Source: CAD feature listing. Evaluate the final solid. Frame: model axes, mm. A direction names the side the tool comes from. Coordinates: 2 decimals unless noted, no trailing zeros. Write each loop counter-clockwise with the first axis right and the second up, starting at its lowest first coordinate (ties: lowest second). Pieces come first, ordered by that corner, then holes. Notation, with made-up numbers: (36.5, -9.75) -> (89.5, -9.75) arc R21 ccw to (89.5, 10.25) -> close; hole circle Ø10 at (-34, 78). An arc over 180 degrees is marked (long way). One line per item, written item: value. Start each with the question number.
1. Mould query, pull axis Y, two halves, no side actions, for faces 3 (the flat face through (-1, 47, -1380)), 4 (the flat face through (1, -50, -1380)), 5 (the flat face through (-48, 0, 0)). Classes: released by +Y, released by -Y, zero draft, split by the parting line, or undercut.
2. First-contact query: P1, Ø1.5, axis at x = 48, z = 41.5, coming from the -Y side. Flat tip, straight axial feed; report the tip coordinate or a pass-through.
3. Section query C-C, the plane x = -18.5. Output: boundary loops of the cut face in (y, z).
4. Access query for faces 1 (the flat face through (49, 1, -2843)), 2 (the flat face through (-47, -1, -1380)). Directions: +Z, -Z, +X, -X, +Y, -Y. A direction counts if a zero-diameter tool reaches every point of the face in a straight line with its end or side. Return the directions, or none.
5. Section query B-B, the plane z = -1213.5. Output: boundary loops of the cut face in (x, y), and give its area (3 significant figures).
6. Section query A-A, the plane y = 20. Output: boundary loops of the cut face in (x, z).
7. Line query: line 1 (Y direction, x = 22, z = -420.5); line 2 (Y direction, x = 44, z = -1473.5). Output: solid intervals per line, ascending.
from build123d import *

# Parameters (mm, degrees)
EXTRUDE_1_DEPTH = 2800
EXTRUDE_2_DEPTH = 3


with BuildPart() as part:
    # Эскиз1 → Бобышка-Вытянуть1 (new body)
    with BuildSketch(Plane.XY):
        with BuildLine():
            Line((-44, 50), (44, 50))
            ThreePointArc((44, 50), (48.242640687, 48.242640687), (50, 44))
            Line((50, 44), (50, -44))
            ThreePointArc((50, -44), (48.242640687, -48.242640687), (44, -50))
            Line((44, -50), (-44, -50))
            ThreePointArc((-44, -50), (-48.242640687, -48.242640687), (-50, -44))
            Line((-50, -44), (-50, 44))
            ThreePointArc((-50, 44), (-48.242640687, 48.242640687), (-44, 50))
        make_face()
        with BuildLine():
            Line((-43, 47), (43, 47))
            ThreePointArc((43, 47), (45.828427125, 45.828427125), (47, 43))
            Line((47, 43), (47, -43))
            ThreePointArc((47, -43), (45.828427125, -45.828427125), (43, -47))
            Line((43, -47), (-43, -47))
            ThreePointArc((-43, -47), (-45.828427125, -45.828427125), (-47, -43))
            Line((-47, -43), (-47, 43))
            ThreePointArc((-47, 43), (-45.828427125, 45.828427125), (-43, 47))
        make_face(mode=Mode.SUBTRACT)
    extrude(amount=-EXTRUDE_1_DEPTH)

    # Эскиз2 → Бобышка-Вытянуть2 (add)
    with BuildSketch(Plane(origin=(50, 0, 0), x_dir=(0, 0, -1), z_dir=(1, 0, 0))):
        Polygon((0, -44), (0, 44), (-88, -44), align=None)
        Polygon((2800, -44), (2800, 44), (2888, -44), align=None)
    extrude(amount=-EXTRUDE_2_DEPTH)


solid = part.part
Computed values:
1. face 3: undercut
1. face 4: released by -Y
1. face 5: zero draft
2. P1: stops at y = -44
3. outline: (-50, -2800) -> (-47, -2800) -> (-47, 0) -> (-50, 0) -> close; (47, -2800) -> (50, -2800) -> (50, 0) -> (47, 0) -> close
4. face 1: -Z, +X, -X, +Y
4. face 2: +Z, -Z
5. outline: (-50, -44) arc R6 ccw to (-44, -50) -> (44, -50) arc R6 ccw to (50, -44) -> (50, 44) arc R6 ccw to (44, 50) -> (-44, 50) arc R6 ccw to (-50, 44) -> close; hole (-47, -43) arc R4 ccw to (-43, -47) -> (43, -47) arc R4 ccw to (47, -43) -> (47, 43) arc R4 ccw to (43, 47) -> (-43, 47) arc R4 ccw to (-47, 43) -> close
5. area: 1,150 mm²
6. outline: (-50, -2800) -> (-47, -2800) -> (-47, 0) -> (-50, 0) -> close; (47, -2824) -> (50, -2824) -> (50, 24) -> (47, 24) -> close
7. line 1: y = -50 to -47, 47 to 50
7. line 2: y = -50 to -46.87, 46.87 to 50
